from build123d import *

# Parameters (mm, degrees)
SKETCH_3_R           = 48
EXTRUDE_2_DEPTH      = 3
SKETCH_4_R           = 3
CUT_EXTRUDE_1_DEPTH  = 3
EXTRUDE_3_DEPTH      = 35
SKETCH_6_R           = 3
SKETCH_6_R_2         = 1.5
CUT_EXTRUDE_2_DEPTH  = 35
SKETCH_7_R           = 1.55
CUT_EXTRUDE_5_DEPTH  = 35
CUT_EXTRUDE_START    = -35
SKETCH_9_R           = 48
SKETCH_9_R_2         = 40
CUT_EXTRUDE_6_DEPTH  = 35
SKETCH_10_R          = 40
CUT_EXTRUDE_7_DEPTH  = 35
SKETCH_11_W          = 111.588244868
SKETCH_11_H          = 82.223617215
CUT_EXTRUDE_8_DEPTH  = 35
SKETCH_12_R          = 1
CUT_EXTRUDE_9_DEPTH  = 35
SKETCH_13_R          = 2.1
CUT_EXTRUDE_10_DEPTH = 35
SKETCH_14_R          = 1.55
CUT_EXTRUDE_11_DEPTH = 35


with BuildPart() as part:
    # 草图3 → 凸台-拉伸2 (new body)
    with BuildSketch(Plane.XY):
        Circle(SKETCH_3_R)
    extrude(amount=EXTRUDE_2_DEPTH)

    # 草图4 → 切除-拉伸1 (cut)
    with BuildSketch(Plane.XY.offset(3)):
        Circle(SKETCH_4_R)
    extrude(amount=-CUT_EXTRUDE_1_DEPTH, mode=Mode.SUBTRACT)

    # 草图5 → 凸台-拉伸3 (add)
    with BuildSketch(Plane.XY.offset(3)):
        with BuildLine():
            ThreePointArc((0, 12.5), (0.146446609, 12.853553391), (0.5, 13))
            Line((0.5, 13), (39.5, 13))
            ThreePointArc((39.5, 13), (39.853553391, 12.853553391), (40, 12.5))
            Line((40, 12.5), (40, -12.5))
            ThreePointArc((40, -12.5), (39.853553391, -12.853553391), (39.5, -13))
            Line((39.5, -13), (0.5, -13))
            ThreePointArc((0.5, -13), (0.146446609, -12.853553391), (0, -12.5))
            Line((0, -12.5), (0, -11.5))
            ThreePointArc((0, -11.5), (0.146446609, -11.146446609), (0.5, -11))
            Line((0.5, -11), (37.5, -11))
            ThreePointArc((37.5, -11), (37.853553391, -10.853553391), (38, -10.5))
            Line((38, -10.5), (38, 0))
            Line((38, 0), (38, 10.5))
            ThreePointArc((38, 10.5), (37.853553391, 10.853553391), (37.5, 11))
            Line((37.5, 11), (0.5, 11))
            ThreePointArc((0.5, 11), (0.146446609, 11.146446609), (0, 11.5))
            Line((0, 11.5), (0, 12.5))
        make_face()
    extrude(amount=EXTRUDE_3_DEPTH)

    # 草图6 → 切除-拉伸2 (cut)
    with BuildSketch(Plane(origin=(40, 0, 0), x_dir=(0, 0, -1), z_dir=(1, 0, 0))):
        with Locations((-25, 0)):
            Circle(SKETCH_6_R)
        with Locations((-20, -5)):
            Circle(SKETCH_6_R_2)
        with Locations((-20, 5)):
            Circle(SKETCH_6_R_2)
        with Locations((-30, -5)):
            Circle(SKETCH_6_R_2)
        with Locations((-30, 5)):
            Circle(SKETCH_6_R_2)
    extrude(amount=-CUT_EXTRUDE_2_DEPTH, mode=Mode.SUBTRACT)

    # 草图7 → 切除-拉伸5 (cut)
    with BuildSketch(Plane.XY.offset(3)):
        with Locations((-35, 0)):
            Circle(SKETCH_7_R)
        with Locations((-24.748737342, 24.748737342)):
            Circle(SKETCH_7_R)
        with Locations((0, 35)):
            Circle(SKETCH_7_R)
        with Locations((24.748737342, 24.748737342)):
            Circle(SKETCH_7_R)
        with Locations((35, 0)):
            Circle(SKETCH_7_R)
        with Locations((24.748737342, -24.748737342)):
            Circle(SKETCH_7_R)
        with Locations((0, -35)):
            Circle(SKETCH_7_R)
        with Locations((-24.748737342, -24.748737342)):
            Circle(SKETCH_7_R)
    extrude(amount=-CUT_EXTRUDE_5_DEPTH, mode=Mode.SUBTRACT)

    # 草图9 → 切除-拉伸6 (cut)
    with BuildSketch(Plane.XY.offset(3).offset(CUT_EXTRUDE_START)):
        Circle(SKETCH_9_R)
        Circle(SKETCH_9_R_2, mode=Mode.SUBTRACT)
    extrude(amount=CUT_EXTRUDE_6_DEPTH, mode=Mode.SUBTRACT)

    # 草图10 → 切除-拉伸7 (cut)
    with BuildSketch(Plane.XY.offset(3)):
        Circle(SKETCH_10_R)
    extrude(amount=CUT_EXTRUDE_7_DEPTH, mode=Mode.SUBTRACT)


with BuildPart() as cut_extrude_7_piece_1:
    # of the separate pieces the step leaves, piece 1, a body of its own (cut_extrude_7_pieces)
    add(part.part.solids().sort_by_distance((40, 0, 0))[0])

    # 草图12 → 切除-拉伸9 (cut)
    with BuildSketch(Plane.XY.offset(3)):
        with BuildLine():
            ThreePointArc((-4, 5), (-5.707106781, 5.707106781), (-5, 4))
            Line((-5, 4), (-5, 5))
            Line((-5, 5), (-4, 5))
        make_face()
        with BuildLine():
            Line((-5, 5), (-5, 4))
            ThreePointArc((-5, 4), (-4.292893219, 4.292893219), (-4, 5))
            Line((-4, 5), (-5, 5))
        make_face()
        with Locations((-5, -5)):
            Circle(SKETCH_12_R)
        with Locations((5, -5)):
            Circle(SKETCH_12_R)
        with Locations((5, 5)):
            Circle(SKETCH_12_R)
    extrude(amount=-CUT_EXTRUDE_9_DEPTH, mode=Mode.SUBTRACT)

    # 草图13 → 切除-拉伸10 (cut)
    with BuildSketch(Plane.XY.offset(3)):
        with Locations((0, 35)):
            Circle(SKETCH_13_R)
        with Locations((24.748737342, 24.748737342)):
            Circle(SKETCH_13_R)
        with Locations((35, 0)):
            Circle(SKETCH_13_R)
        with Locations((24.748737342, -24.748737342)):
            Circle(SKETCH_13_R)
        with Locations((0, -35)):
            Circle(SKETCH_13_R)
        with Locations((-24.748737342, -24.748737342)):
            Circle(SKETCH_13_R)
        with Locations((-35, 0)):
            Circle(SKETCH_13_R)
        with Locations((-24.748737342, 24.748737342)):
            Circle(SKETCH_13_R)
    extrude(amount=-CUT_EXTRUDE_10_DEPTH, mode=Mode.SUBTRACT)

    # 草图14 → 切除-拉伸11 (cut)
    with BuildSketch(Plane.XY.offset(3)):
        with Locations((-5, 5)):
            Circle(SKETCH_14_R)
        with Locations((5, 5)):
            Circle(SKETCH_14_R)
        with Locations((5, -5)):
            Circle(SKETCH_14_R)
        with Locations((-5, -5)):
            Circle(SKETCH_14_R)
    extrude(amount=-CUT_EXTRUDE_11_DEPTH, mode=Mode.SUBTRACT)


with BuildPart() as cut_extrude_7_piece_2:
    # of the separate pieces the step leaves, piece 2, a body of its own (cut_extrude_7_pieces)
    add(part.part.solids().sort_by_distance((40, -12.5, 3))[0])


with BuildPart() as cut_extrude_7_piece_3:
    # of the separate pieces the step leaves, piece 3, a body of its own (cut_extrude_7_pieces)
    add(part.part.solids().sort_by_distance((39.5, 13, 3))[0])


with BuildPart() as cut_extrude_8_tool:
    # 草图11 → 切除-拉伸8 (new body)
    with BuildSketch(Plane(origin=(40, 0, 0), x_dir=(0, 0, -1), z_dir=(1, 0, 0))):
        with Locations((-58.794122434, 24.320721942)):
            Rectangle(SKETCH_11_W, SKETCH_11_H)
    extrude(amount=-CUT_EXTRUDE_8_DEPTH)


with BuildPart() as cut_extrude_7_piece_2_1:
    add(cut_extrude_7_piece_2.part)

    # 切除-拉伸8: cut by cut_extrude_8_tool
    add(cut_extrude_8_tool.part, mode=Mode.SUBTRACT)


with BuildPart() as cut_extrude_7_piece_3_1:
    add(cut_extrude_7_piece_3.part)

    # 切除-拉伸8: cut by cut_extrude_8_tool
    add(cut_extrude_8_tool.part, mode=Mode.SUBTRACT)


solid = cut_extrude_7_piece_1.part
For this review, take the finished solid that the model builds, in its own axes (mm). Round coordinates to 2 decimals unless told otherwise and drop trailing zeros. Loops run counter-clockwise (first coordinate to the right, second up) from the corner with the lowest first, then second, coordinate; pieces in that order, holes last. Notation, with made-up numbers: (-26, 72.25) - (32, 72.25) arc R13 ccw to (32, 92.25) - close; hole circle Ø7 at (88, 12.25). An arc over 180 degrees is marked (long way). Use one line per item in the form item = value.
Item 1: Mouldability with a two-part tool opening along X and no side actions: class faces 1 (the flat face through (8, 1, 3)), 2 (the cylindrical face through (-6.55, 5.07, 1.52)), 3 (the cylindrical face through (-8.67, -39.05, 1.48)) as +X half, -X half, draft (parallel to the pull), parting line (faces both ways), or undercut.
Answers:
face_1 = draft
face_2 = undercut
face_3 = parting line
Item 2: For line 1 (Y direction, x = 0, z = 2.4); line 2 (Y direction, x = -6, z = 1.9); line 3 (Y direction, x = -5, z = 1.25), list the stretches that pass through material, from the lowest coordinate up.
Answers:
line_1 = -40 to -37.1, -32.9 to -3, 3 to 32.9, 37.1 to 40
line_2 = -39.55 to -6.18, -3.82 to 3.82, 6.18 to 39.55
line_3 = -39.69 to -6.55, -3.45 to 3.45, 6.55 to 39.69
Item 3: Consider section D-D on x = 35. Write out the cut boundary in (y, z), then the cut area to 3 significant figures.
Answers:
outline = (-19.36, 0) - (-2.1, 0) - (-2.1, 3) - (-19.36, 3) - close; (2.1, 0) - (19.36, 0) - (19.36, 3) - (2.1, 3) - close
area = 104 mm^2
Item 4: Consider section C-C on z = 2.05. State how many separate pieces and enclosed holes the cut face has, then the cut area to 3 significant figures.
Answers:
separate_pieces = 1
enclosed_holes = 13
area = 4,860 mm^2
Item 5: Consider section B-B on x = 5. Write out the cut boundary in (y, z).
Answers:
outline = (-39.69, 0) - (-6.55, 0) - (-6.55, 3) - (-39.69, 3) - close; (-3.45, 0) - (3.45, 0) - (3.45, 3) - (-3.45, 3) - close; (6.55, 0) - (39.69, 0) - (39.69, 3) - (6.55, 3) - close
Item 6: Clearance check with flat-ended pins moving along their axes: P1, Ø5.5, axis at x = 0, y = 0, coming from the +Z side; P2, Ø1.5, axis at y = 6, z = 2.5, coming from the -X side. State where each tip first meets the part, or that it passes through.
Answers:
P1 = through
P2 = -39.65
Item 7: Consider section A-A on y = 0. Write out the cut boundary in (x, z).
Answers:
outline = (-40, 0) - (-37.1, 0) - (-37.1, 3) - (-40, 3) - close; (-32.9, 0) - (-3, 0) - (-3, 3) - (-32.9, 3) - close; (3, 0) - (32.9, 0) - (32.9, 3) - (3, 3) - close; (37.1, 0) - (40, 0) - (40, 3) - (37.1, 3) - close
